```python
from build123d import *
from build123d.topology import SkipClean

# Parameters (mm, degrees)
SKETCH2_R           = 7.5
BOSS_EXTRUDE1_DEPTH = 10
FILLET1_R           = 5
BOSS_EXTRUDE2_START = -24
SKETCH3_R           = 11
SKETCH3_R_2         = 7.5
BOSS_EXTRUDE2_DEPTH = 24
CUT_EXTRUDE1_REACH  = 135.566
SKETCH4_R           = 1.55
SKETCH6_W           = 37.11251069
SKETCH6_H           = 1
CUT_EXTRUDE3_DEPTH  = 10
SKETCH7_W           = 36.737317401
SKETCH7_H           = 1
CUT_EXTRUDE4_DEPTH  = 3
FILLET2_R           = 5
SKETCH9_W           = 0.416349778
SKETCH9_H           = 0.714723325
CUT_EXTRUDE6_DEPTH  = 1
SKETCH8_R           = 1.5
CUT_EXTRUDE5_DEPTH  = 7


with BuildPart() as part:
    # Sketch2 → Boss-Extrude1 (new body)
    with BuildSketch(Plane.XY):
        with BuildLine():
            Line((-22.5, 3.831552556), (-22.5, 14.831552556))
            Line((-22.5, 14.831552556), (-12.5, 14.831552556))
            Line((-12.5, 14.831552556), (-12.5, 3.831552556))
            Line((-12.5, 3.831552556), (-2.5, 3.831552556))
            Line((-2.5, 3.831552556), (-2.5, 14.831552556))
            Line((-2.5, 14.831552556), (7.5, 14.831552556))
            Line((7.5, 14.831552556), (7.5, 3.831552556))
            Line((7.5, 3.831552556), (88.192235936, 3.831552556))
            ThreePointArc((88.192235936, 3.831552556), (91.819805392, 9.932478429), (98.5, 12.331552556))
            ThreePointArc((98.5, 12.331552556), (109, 1.831552556), (98.5, -8.668447444))
            Line((98.5, -8.668447444), (-98.5, -8.668447444))
            ThreePointArc((-98.5, -8.668447444), (-109, 1.831552556), (-98.5, 12.331552556))
            ThreePointArc((-98.5, 12.331552556), (-91.358571571, 9.975203317), (-87.021759717, 3.831552556))
            Line((-87.021759717, 3.831552556), (-22.5, 3.831552556))
        make_face()
        with Locations((-98.5, 1.831552556)):
            Circle(SKETCH2_R, mode=Mode.SUBTRACT)
        with Locations((98.5, 1.831552556)):
            Circle(SKETCH2_R, mode=Mode.SUBTRACT)
    extrude(amount=BOSS_EXTRUDE1_DEPTH)

    # Fillet1
    fillet1_edges = [part.edges().sort_by_distance(p)[0] for p in [
        (88.192235936, 3.831552556, 5),
    ]]
    fillet(fillet1_edges, radius=FILLET1_R)

    # Sketch3 → Boss-Extrude2 (add)
    with BuildSketch(Plane.XY.offset(10).offset(BOSS_EXTRUDE2_START)):
        with Locations((-98.5, 1.831552556)):
            Circle(SKETCH3_R)
        with Locations((-98.5, 1.831552556)):
            Circle(SKETCH3_R_2, mode=Mode.SUBTRACT)
    boss_extrude2 = extrude(amount=BOSS_EXTRUDE2_DEPTH)

    # Mirror1: Boss-Extrude2 across plane
    with SkipClean():  # the faces are left unmerged after this step: merging them gives an invalid solid
        add(boss_extrude2.mirror(Plane(origin=(0, 0, 0), x_dir=(0, 0, 1), z_dir=(1, 0, 0))))

    # Cut-Extrude1: up to this face of the body (flat: up to its plane)
    cut_extrude1_end = Plane(part.part.faces().sort_by_distance((7.5, 9.331552556, 5))[0])
    # Sketch4 → Cut-Extrude1 (cut, up to the picked face)
    with BuildSketch(Plane.ZY.offset(22.5), mode=Mode.PRIVATE) as cut_extrude1_sk1:
        with Locations((5, 10.805752832)):
            Circle(SKETCH4_R)
    cut_extrude1_tool1 = split(extrude(cut_extrude1_sk1.sketch, amount=-CUT_EXTRUDE1_REACH, mode=Mode.PRIVATE), bisect_by=cut_extrude1_end, keep=Keep.BOTH, mode=Mode.PRIVATE)
    add(cut_extrude1_tool1.solids().sort_by(Axis((-22.5, 10.805753, 5), (1, 0, 0)))[0], mode=Mode.SUBTRACT)

    # Sketch6 → Cut-Extrude3 (cut)
    with BuildSketch(Plane(origin=(110, 0, 0), x_dir=(0, 0, -1), z_dir=(1, 0, 0))):
        with Locations((1.381927251, 1.831552556)):
            Rectangle(SKETCH6_W, SKETCH6_H)
    cut_extrude3 = extrude(amount=-CUT_EXTRUDE3_DEPTH, mode=Mode.SUBTRACT)

    # Mirror2: Cut-Extrude3 across plane
    add(cut_extrude3.mirror(Plane(origin=(0, 0, 0), x_dir=(0, 0, 1), z_dir=(1, 0, 0))), mode=Mode.SUBTRACT)

    # Sketch7 → Cut-Extrude4 (cut)
    with BuildSketch(Plane(origin=(0, 14.831552556, 0), x_dir=(1, 0, 0), z_dir=(0, 1, 0))):
        with Locations((-7.879171978, -4.654369626)):
            Rectangle(SKETCH7_W, SKETCH7_H)
    extrude(amount=-CUT_EXTRUDE4_DEPTH, mode=Mode.SUBTRACT)

    # Fillet2
    fillet2_edges = [part.edges().sort_by_distance(p)[0] for p in [
        (-87.021759717, 3.831552556, 5),
    ]]
    fillet(fillet2_edges, radius=FILLET2_R)

    # Sketch9 → Cut-Extrude6 (cut)
    with BuildSketch(Plane(origin=(0, 3.831552556, 0), x_dir=(1, 0, 0), z_dir=(0, 1, 0))):
        with Locations((-81.24394575, -5.497333598)):
            Rectangle(SKETCH9_W, SKETCH9_H)
    extrude(amount=-CUT_EXTRUDE6_DEPTH, mode=Mode.SUBTRACT)

    # Sketch8 → Cut-Extrude5 (cut)
    with BuildSketch(Plane(origin=(0, 3.831552556, 0), x_dir=(1, 0, 0), z_dir=(0, 1, 0))):
        with Locations(Location((-66.24976189, -5, 0), (0, 0, 270))):
            Circle(SKETCH8_R)
        with Locations(Location((-54.24976189, -5, 0), (0, 0, 270))):
            Circle(SKETCH8_R)
        with Locations(Location((-32.502764064, -5, 0), (0, 0, 270))):
            Circle(SKETCH8_R)
        with Locations(Location((32.497235936, -5, 0), (0, 0, 270))):
            Circle(SKETCH8_R)
        with Locations(Location((54.25023811, -5, 0), (0, 0, 270))):
            Circle(SKETCH8_R)
        with Locations(Location((66.25023811, -5, 0), (0, 0, 270))):
            Circle(SKETCH8_R)
    extrude(amount=-CUT_EXTRUDE5_DEPTH, mode=Mode.SUBTRACT)


solid = part.part
```
The listing builds one solid part. Answer for the finished solid, in the listing's coordinates (mm). A direction names the side the tool comes from. Give positions to 0.01 mm unless a question says otherwise; leave off trailing zeros. Order: outer loops, then holes, each group sorted by start corner. A loop starts at its lowest first (then second) coordinate and runs counter-clockwise, first axis right, second up.
Item 1: For a pull along Y with two mould halves and no side action, classify faces 1 (the face through (108, 2.332, -2)), 2 (the face through (-91, 0, -14)), 3 (the face through (-108, 1.332, -2)), 4 (the face through (-18, 14.832, 8)) as pulls with the +Y half, pulls with the -Y half, needs draft (parallel to the pull), parting line crosses it, or undercut.
From the geometry:
face 1: undercut
face 2: needs draft
face 3: undercut
face 4: pulls with the +Y half
Item 2: The part is cut by section D-D, the plane x = -28. Give the vertices of the cut face in (y, z), and give its area (3 significant figures).
From the geometry:
outline: (-8.67, 0) - (3.83, 0) - (3.83, 10) - (-8.67, 10) - close
area: 125 mm2
Item 3: Find the intervals of material crossed by probe 1 along X at (y, z) = (2.5, 7.5); probe 2 along Y at (x, z) = (98.5, -2.25); probe 3 along X at (y, z) = (5.25, 3), in increasing order.
From the geometry:
probe 1: x = -109.48 to -105.97, -91.03 to 91.03, 105.97 to 109.48
probe 2: y = -9.17 to -5.67, 9.33 to 12.83
probe 3: x = -108.96 to -105.18, -91.82 to -87.27, -22.5 to -12.5, -2.5 to 7.5, 88.04 to 91.82, 105.18 to 108.96
Item 4: The part is cut by section A-A, the plane z = -9.25. Give the vertices of the cut face in (x, y), and give its area (3 significant figures).
From the geometry:
outline: (-109.49, 1.33) arc R11 ccw (long way) to (-109.49, 2.33) - (-105.98, 2.33) arc R7.5 cw (long way) to (-105.98, 1.33) - close; (105.98, 1.33) arc R7.5 cw (long way) to (105.98, 2.33) - (109.49, 2.33) arc R11 ccw (long way) to (109.49, 1.33) - close
area: 400 mm2
Item 5: Given pin 1 Ø0.9 at (x, z) = (65.5, 5.5) entering from +Y; pin 2 Ø3.5 at (x, z) = (-33, 5.5) entering from +Y; pin 3 Ø2.5 at (y, z) = (10.81, 5) entering from -X, each flat-ended and moving along its own axis, determine where each tip first touches the part or whether it passes through.
From the geometry:
pin 1: stops at y = -3.17
pin 2: stops at y = 3.83
pin 3: stops at x = -106.33
Item 6: The part is cut by section C-C, the plane x = 0. Give the vertices of the cut face in (y, z), and give its area (3 significant figures).
From the geometry:
outline: (-8.67, 0) - (14.83, 0) - (14.83, 4.15) - (12.1, 4.15) arc R1.55 cw (long way) to (12.35, 5.15) - (14.83, 5.15) - (14.83, 10) - (-8.67, 10) - close
area: 225 mm2
Item 7: Which of the six approach directions +Z, -Z, +X, -X, +Y, -Y give full straight-line access (tool end or side, diameter ignored) to faces 5 (the face through (-54, 3.832, 3)), 6 (the face through (-108, 2.332, -2)), 7 (the face through (108.486, 6.445, -2.168))?
From the geometry:
face 5: +Z, -Z, +Y
face 6: +Z, -Z, -X
face 7: -Z
Item 8: The part is cut by section B-B, the plane x = 98.5. Give the vertices of the cut face in (y, z), and give its area (3 significant figures).
From the geometry:
outline: (-9.17, -14) - (-5.67, -14) - (-5.67, 10) - (-9.17, 10) - close; (9.33, -14) - (12.83, -14) - (12.83, 10) - (9.33, 10) - close
area: 168 mm2
